```python
from build123d import *

# Parameters (mm, degrees)
SKETCH_1_R          = 7.5
EXTRUDE_1_DEPTH     = 5
SKETCH_2_R          = 5
CUT_EXTRUDE_1_DEPTH = 2
SKETCH_3_R          = 3.4
CUT_EXTRUDE_2_DEPTH = 12.022703843
SKETCH_4_W          = 7.409830056
SKETCH_4_H          = 10
EXTRUDE_3_DEPTH     = 5
SKETCH_5_W          = 3
SKETCH_5_H          = 10
EXTRUDE_4_DEPTH     = 6
SKETCH_6_R          = 1
CUT_EXTRUDE_3_DEPTH = 30.210443338


with BuildPart() as part:
    # 草图1 → 凸台-拉伸1 (new body)
    with BuildSketch(Plane(origin=(0, 0, 0), x_dir=(0, 0, -1), z_dir=(1, 0, 0))):
        Circle(SKETCH_1_R)
    extrude(amount=EXTRUDE_1_DEPTH)

    # 草图2 → 切除-拉伸1 (cut)
    with BuildSketch(Plane(origin=(5, 0, 0), x_dir=(0, 0, -1), z_dir=(1, 0, 0))):
        Circle(SKETCH_2_R)
    extrude(amount=-CUT_EXTRUDE_1_DEPTH, mode=Mode.SUBTRACT)

    # 草图3 → 切除-拉伸2 (cut, through all)
    with BuildSketch(Plane(origin=(3, 0, 0), x_dir=(0, 0, -1), z_dir=(1, 0, 0))):
        Circle(SKETCH_3_R)
    extrude(amount=-CUT_EXTRUDE_2_DEPTH, mode=Mode.SUBTRACT)

    # 草图4 → 凸台-拉伸3 (add)
    with BuildSketch(Plane(origin=(5, 0, 0), x_dir=(0, 0, -1), z_dir=(1, 0, 0))):
        with Locations((9.295084972, 0)):
            Rectangle(SKETCH_4_W, SKETCH_4_H)
        with Locations((-9.295084972, 0)):
            Rectangle(SKETCH_4_W, SKETCH_4_H)
    extrude(amount=-EXTRUDE_3_DEPTH)

    # 草图5 → 凸台-拉伸4 (add)
    with BuildSketch(Plane(origin=(5, 0, 0), x_dir=(0, 0, -1), z_dir=(1, 0, 0))):
        with Locations((11.5, 0)):
            Rectangle(SKETCH_5_W, SKETCH_5_H)
        with Locations((-11.5, 0)):
            Rectangle(SKETCH_5_W, SKETCH_5_H)
    extrude(amount=EXTRUDE_4_DEPTH)

    # 草图6 → 切除-拉伸3 (cut, through all)
    with BuildSketch(Plane(origin=(0, 0, -13), x_dir=(-1, 0, 0), z_dir=(0, 0, -1))):
        with Locations((-8.5, 0)):
            Circle(SKETCH_6_R)
    extrude(amount=-CUT_EXTRUDE_3_DEPTH, mode=Mode.SUBTRACT)


solid = part.part
```
Check sheet for the modelled part. Datum: model origin and axes. Units: mm. A direction names the side the tool comes from. Give positions to 0.01 mm unless a question says otherwise; leave off trailing zeros. Write each loop counter-clockwise with the first axis right and the second up, starting at its lowest first coordinate (ties: lowest second). Pieces come first, ordered by that corner, then holes. Notation, with made-up numbers: (24.25, 23.25) - (63.25, 23.25) arc R9 cw to (63.25, 29.25) - close; hole circle Ø9 at (-29.75, -23.5). An arc over 180 degrees is marked (long way). Answer as a JSON object with one key per item and string values. Group by question number.
1) Sectioned sample at A-A (z = 0). Record the cut outline in (x, y).
2) Thickness scan on probe 1 along Y at (x, z) = (1.65, 0); probe 2 along Y at (x, z) = (8.5, 12.05); probe 3 along Z at (x, y) = (6, -2.25). Record the ranges inside material, lowest first. Write a range as from..to.
3) Depth check by flat-ended pin: P1, Ø6, axis at x = 6.5, z = -11, coming from the +Y side; P2, Ø2, axis at y = 4, z = 2.5, coming from the +X side; P3, Ø6, axis at x = 5.5, z = -7.5, coming from the -Y side. Enter the tip coordinate at first touch or a pass-through.
4) Sectioned sample at D-D (z = -11). Record the cut outline in (x, y).
5) Sectioned sample at B-B (x = 8.5). Record the cut outline in (y, z), then the cut area to 3 significant figures.
6) Access from +Z, -Z, +X, -X, +Y, -Y to the whole of each face (thin tool, end or side, straight path). Record for faces 1 (the face through (4, -5, -10)), 2 (the face through (4, 5, 10)), 3 (the face through (7, 0, 10)).
7) Sectioned sample at C-C (y = 0). Record the cut outline in (x, z).
8) Release check for a two-part mould opening along Y. For faces 4 (the face through (4, -5, 10)), 5 (the face through (4, 5, -10)), 6 (the face through (0, -2, 3)), 7 (the face through (1.52, -3.32, 0.74)) record: pulls with the +Y half, pulls with the -Y half, needs draft (parallel to the pull), parting line crosses it, or undercut.
Geometry results:
{
 "1": {"outline": "(0, -7.5) - (5, -7.5) - (5, -5) - (3, -5) - (3, -3.4) - (0, -3.4) - close; (0, 3.4) - (3, 3.4) - (3, 5) - (5, 5) - (5, 7.5) - (0, 7.5) - close"},
 "2": {"probe 1": "y = -7.5..-3.4, 3.4..7.5", "probe 2": "y = -5..-1, 1..5", "probe 3": "z = -13..-10, 10..13"},
 "3": {"P1": "stops at y = 5", "P2": "stops at x = 5", "P3": "stops at y = -5.97"},
 "4": {"outline": "(0, -5) - (11, -5) - (11, 5) - (0, 5) - close; hole circle Ø2 at (8.5, 0)"},
 "5": {"outline": "(-5, -13) - (-1, -13) - (-1, -10) - (-5, -10) - close; (-5, 10) - (-1, 10) - (-1, 13) - (-5, 13) - close; (1, -13) - (5, -13) - (5, -10) - (1, -10) - close; (1, 10) - (5, 10) - (5, 13) - (1, 13) - close", "area": "48.0 mm^2"},
 "6": {"face 1": "-Z, +X, -X, -Y", "face 2": "+Z, +X, -X, +Y", "face 3": "+X, +Y, -Y"},
 "7": {"outline": "(0, -13) - (7.5, -13) - (7.5, -10) - (5, -10) - (5, -5) - (3, -5) - (3, -3.4) - (0, -3.4) - close; (0, 3.4) - (3, 3.4) - (3, 5) - (5, 5) - (5, 10) - (7.5, 10) - (7.5, 13) - (0, 13) - close; (9.5, -13) - (11, -13) - (11, -10) - (9.5, -10) - close; (9.5, 10) - (11, 10) - (11, 13) - (9.5, 13) - close"},
 "8": {"face 4": "pulls with the -Y half", "face 5": "pulls with the +Y half", "face 6": "needs draft", "face 7": "undercut"}
}
